Check sheet for the modelled part. Datum: model origin and axes. Units: mm. A direction names the side the tool comes from. Coordinates: 2 decimals unless noted, no trailing zeros. Order: outer loops, then holes, each group sorted by start corner. A loop starts at its lowest first (then second) coordinate and runs counter-clockwise, first axis right, second up. Notation, with made-up numbers: M 27,16.5 L 51,16.5 A30 cw 51,55.5 Z; hole C 44,-10.5 d1. An arc over 180 degrees is marked long. Answer in a Markdown table with one row per item. Add a question column.
from build123d import *

# Parameters (mm, degrees)
SKETCH1_W           = 60
SKETCH1_H           = 32
BOSS_EXTRUDE1_DEPTH = 2
BOSS_EXTRUDE2_DEPTH = 6
SKETCH3_W           = 10
SKETCH3_H           = 32
BOSS_EXTRUDE3_DEPTH = 2


with BuildPart() as part:
    # Sketch1 → Boss-Extrude1 (new body)
    with BuildSketch(Plane(origin=(0, 0, 0), x_dir=(1, 0, 0), z_dir=(0, 1, 0))):
        Rectangle(SKETCH1_W, SKETCH1_H)
    extrude(amount=BOSS_EXTRUDE1_DEPTH)

    # Sketch2 → Boss-Extrude2 (add)
    with BuildSketch(Plane.XZ):
        Polygon((-30, -18), (32, -18), (32, 18), (-30, 18), (-30, 16), (30, 16), (30, -16), (-30, -16), align=None)
    extrude(amount=-BOSS_EXTRUDE2_DEPTH)

    # Sketch3 → Boss-Extrude3 (add)
    with BuildSketch(Plane.XZ):
        with Locations((-35, 0)):
            Rectangle(SKETCH3_W, SKETCH3_H)
    extrude(amount=-BOSS_EXTRUDE3_DEPTH)


solid = part.part
1. Release check for a two-part mould opening along Z. For faces 1 (the flat face through (1, 3, -18)), 2 (the flat face through (32, 3, 0)), 3 (the flat face through (30, 4, 0)), 4 (the flat face through (0, 4, -16)) record: released by +Z, released by -Z, zero draft, split by the parting line, or undercut.
2. Scan lines: line 1 (Z direction, x = 6, y = 3.6); line 2 (X direction, y = 3.8, z = -1.5); line 3 (Y direction, x = 21, z = 4.5). Record each from-to range of solid material in increasing order.
3. Section check A-A on x = -28. Enter the section's corners in (y, z).
4. Set-up check for faces 5 (the flat face through (-30, 3, 17)), 6 (the flat face through (-30, 3, -17)), 7 (the flat face through (0, 4, 16)): record each of +Z, -Z, +X, -X, +Y, -Y from which the full face is reachable in a straight line by a thin tool's end or side.
5. Go/stop test with flat-tipped pins: pin 1 Ø1 at (x, y) = (-35.5, 1) entering from +Z; pin 2 Ø2 at (x, y) = (-37, 0.5) entering from -Z; pin 3 Ø1 at (y, z) = (3, 17) entering from -X. Record where each tip stops, or that it passes through.
6. Section check B-B on y = 4.95. Enter the section's corners in (x, z).
7. Section check C-C on z = -0.5. Enter the section's corners in (x, y), then the cut area to 3 significant figures.
Result sheet:
| question | item | result |
|---|---|---|
| 1 | face 1 | released by -Z |
| 1 | face 2 | zero draft |
| 1 | face 3 | undercut |
| 1 | face 4 | undercut |
| 2 | line 1 | -18 to -16, 16 to 18 |
| 2 | line 2 | 30 to 32 |
| 2 | line 3 | 0 to 2 |
| 3 | outline | M 0,-18 L 6,-18 L 6,-16 L 2,-16 L 2,16 L 6,16 L 6,18 L 0,18 Z |
| 4 | face 5 | +Z, -X, +Y, -Y |
| 4 | face 6 | -Z, -X, +Y, -Y |
| 4 | face 7 | -X, +Y |
| 5 | pin 1 | z = 16 |
| 5 | pin 2 | z = -16 |
| 5 | pin 3 | x = -30 |
| 6 | outline | M -30,-18 L 32,-18 L 32,18 L -30,18 L -30,16 L 30,16 L 30,-16 L -30,-16 Z |
| 7 | outline | M -40,0 L 32,0 L 32,6 L 30,6 L 30,2 L -40,2 Z |
| 7 | area | 152 mm^2 |
